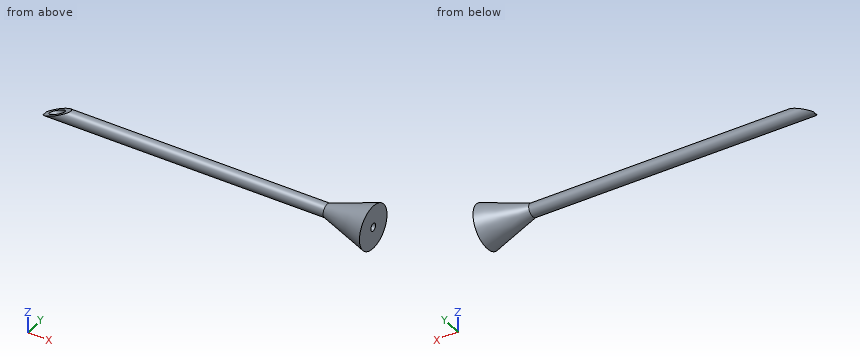
from build123d import *

# Parameters (mm, degrees)
F2_R     = 0.3
F3_DEPTH = 15
F5_DEPTH = 25
F6_DEPTH = 25
F7_R     = 0.175
F8_DEPTH = 25


with BuildPart() as f1:
    # F0 (on Front) → F1 (revolve)
    with BuildSketch(Plane.XZ):
        Polygon((-3, 0), (0, 0), (0, 1), align=None)
    revolve(axis=Axis((-1.5, 0, 0), (-1, 0, 0)))

    # F2 (on Right) → F3 (join)
    with BuildSketch(Plane.YZ):
        Circle(F2_R)
    extrude(amount=-F3_DEPTH)

    # F4 (on Front) → F5 (cut)
    with BuildSketch(Plane.XZ):
        Polygon((-15.222519, 0.32419), (-15.002024, -0.277158), (-13.739192, 0.32419), align=None)
    extrude(amount=-F5_DEPTH, mode=Mode.SUBTRACT)

    # F4 (on Front) → F6 (cut)
    with BuildSketch(Plane.XZ):
        Polygon((-15.222519, 0.32419), (-15.002024, -0.277158), (-13.739192, 0.32419), align=None)
    extrude(amount=F6_DEPTH, mode=Mode.SUBTRACT)

    # F7 (on face) → F8 (cut)
    with BuildSketch(Plane.YZ):
        Circle(F7_R)
    extrude(amount=-F8_DEPTH, mode=Mode.SUBTRACT)


solid = f1.part
The listing builds one solid part. Answer for the finished solid, in the listing's coordinates (mm). Give positions to 0.01 mm unless a question says otherwise; leave off trailing zeros. Write each loop counter-clockwise with the first axis right and the second up, starting at its lowest first coordinate (ties: lowest second). Pieces come first, ordered by that corner, then holes. Notation, with made-up numbers: (41, 63) - (95, 63) arc R4 cw to (95, 68) - close; hole circle Ø5 at (54.5, -36.75). An arc over 180 degrees is marked (long way). Use a Markdown table: item, result.
1. Each of these flat-tipped pins is pushed along its axis until it touches: P1, Ø1, axis at x = -13.5, y = 0, coming from the -Z side; P2, Ø1, axis at x = -2, y = 0, coming from the -Z side. Where does it stop, or does it pass through?
Values follow:
| item | result |
|---|---|
| P1 | stops at z = -0.3 |
| P2 | stops at z = -0.5 |
2. Section A-A on z = 0 is taken. Write down the section's boundary in (x, y) (3 decimals), plus the area to 4 significant figures.
Values follow:
| item | result |
|---|---|
| outline | (-14.42, -0.3) - (-2.1, -0.3) - (0, -1) - (0, -0.175) - (-14.42, -0.175) - close; (-14.42, 0.175) - (0, 0.175) - (0, 1) - (-2.1, 0.3) - (-14.42, 0.3) - close |
| area | 5.075 mm² |
3. Section B-B on x = -5.5 is taken. Write down the section's boundary in (y, z) (3 decimals), plus the area to 3 significant figures.
Values follow:
| item | result |
|---|---|
| outline | circle Ø0.6 at (0, 0); hole circle Ø0.35 at (0, 0) |
| area | 0.187 mm² |
4. Find the intervals of material crossed by probe 1 along Y at (x, z) = (-0.75, -0.3); probe 2 along X at (y, z) = (0.5, -0.7); probe 3 along X at (y, z) = (-0.6, 0.65), in increasing order. Write a range as from..to.
Values follow:
| item | result |
|---|---|
| probe 1 | y = -0.69..0.69 |
| probe 2 | x = -0.42..0 |
| probe 3 | x = -0.35..0 |
